```python
from build123d import *

# Parameters (mm, degrees)
BOSS_EXTRUDE1_DEPTH    = 225
CONVERT_SOLID1_START   = -225
CONVERT_SOLID1_DEPTH   = 450
CONVERT_SOLID1_2_DEPTH = 450


# Read off the part's stored shape, not the designer's step: Convert-Solid1
with BuildPart() as part:
    # Sketch1 → Boss-Extrude1 (new, symmetric)
    with BuildSketch(Plane.XY):
        Polygon((0, 0), (0, 110), (17, 110), (17, 108), (2, 108), (2, 0), align=None)
    extrude(amount=BOSS_EXTRUDE1_DEPTH, both=True)

    # Convert-Solid1 outline → Convert-Solid1 (cut)
    with BuildSketch(Plane.XY.offset(CONVERT_SOLID1_START)):
        with BuildLine():
            ThreePointArc((0, 106), (1.171572875, 108.828427125), (4, 110))
            Line((4, 110), (0, 110))
            Line((0, 110), (0, 106))
        make_face()
    extrude(amount=CONVERT_SOLID1_DEPTH, mode=Mode.SUBTRACT)

    # Convert-Solid1 2 outline → Convert-Solid1 2 (add)
    with BuildSketch(Plane.XY.offset(CONVERT_SOLID1_START)):
        with BuildLine():
            ThreePointArc((2, 106), (2.585786438, 107.414213562), (4, 108))
            Line((4, 108), (2, 108))
            Line((2, 108), (2, 106))
        make_face()
    extrude(amount=CONVERT_SOLID1_2_DEPTH)


solid = part.part
```
Here's how the part is built. I have some questions about the finished solid (model axes, mm). A direction names the side the tool comes from. Coordinates: 2 decimals unless noted, no trailing zeros. Loops run counter-clockwise (first coordinate to the right, second up) from the corner with the lowest first, then second, coordinate; pieces in that order, holes last. Notation, with made-up numbers: M 9.25,-36.5 L 21.25,-36.5 A14 cw 21.25,-22.5 Z; hole C 41.25,68.25 d9. An arc over 180 degrees is marked long. One line per item, written item: value.
1. Please list where these lines run through material, in increasing order: probe 1 along Y at (x, z) = (7.5, -165.5); probe 2 along X at (y, z) = (15.5, -19); probe 3 along Y at (x, z) = (3, 200).
Geometry says:
probe 1: y = 108 to 110
probe 2: x = 0 to 2
probe 3: y = 107.73 to 109.87
2. Will these pins go through, and if not, where does the flat tip stop? pin 1 Ø6.5 at (x, z) = (8.5, 54) entering from -Y; pin 2 Ø4 at (x, y) = (5, 64.5) entering from -Z; pin 3 Ø8 at (y, z) = (40.5, -159.5) entering from +X.
Geometry says:
pin 1: stops at y = 108
pin 2: passes through
pin 3: stops at x = 2
3. On a 3-axis mill with a long thin cutter (end or side, diameter ignored), from which of +Z, -Z, +X, -X, +Y, -Y can I reach the whole of each face in a straight line? I mean faces 1 (the flat face through (2, 54, 3)), 2 (the flat face through (1.5, 67.5, -225)). Say none if no direction works.
Geometry says:
face 1: +Z, -Z, +X, -Y
face 2: -Z, +X, -X, +Y, -Y
4. Imagine slicing it at B-B (y = 71.5). List the corners of the cut face in (x, z) for me.
Geometry says:
outline: M 0,-225 L 2,-225 L 2,225 L 0,225 Z
5. Imagine slicing it at C-C (x = 9.75). List the corners of the cut face in (y, z) for me, and give its area (3 significant figures).
Geometry says:
outline: M 108,-225 L 110,-225 L 110,225 L 108,225 Z
area: 900 mm2
6. Imagine slicing it at A-A (z = -23.5). List the corners of the cut face in (x, y) for me.
Geometry says:
outline: M 0,0 L 2,0 L 2,106 A2 cw 4,108 L 17,108 L 17,110 L 4,110 A4 ccw 0,106 Z
